Design review of the part built by this model. Coordinates are the model's own, in mm. Coordinates: 2 decimals unless noted, no trailing zeros. Write each loop counter-clockwise with the first axis right and the second up, starting at its lowest first coordinate (ties: lowest second). Pieces come first, ordered by that corner, then holes. Notation, with made-up numbers: (6, 82.25) -> (51, 82.25) arc R14 cw to (51, 109.25) -> close; hole circle Ø1 at (30, 88.25). An arc over 180 degrees is marked (long way). Return JSON: item names as keys, results as strings. Group by question number.
Autodesk Inventor part; units mm, degrees
ref_plane "YZ Plane" through (0, 0, 0) normal (1, 0, 0) x (0, 1, 0)
ref_plane "XZ Plane" through (0, 0, 0) normal (0, 1, 0) x (-1, 0, 0)
ref_plane "XY Plane" through (0, 0, 0) normal (0, 0, 1) x (1, 0, 0)
sketch "Boceto1" plane through (0, 0, 0) normal (0, 1, 0) x (-1, 0, 0)
  line L0 (0, 0) -> (80, 0)
  line L1 (80, 0) -> (80, 35)
  line L2 (80, 35) -> (0, 35)
  line L3 (0, 35) -> (0, 0)
  line L4 (75, 35) -> (5, 35)
  line L5 (5, 35) -> (5, 5)
  line L6 (5, 5) -> (75, 5)
  line L7 (75, 5) -> (75, 35)
  dimension "d0" = 80
  dimension "d1" = 35
  dimension "d2" = 70
  dimension "d3" = 30
  dimension "d14" = 5
extrude "Extrusión1" add sketch "Boceto1" along normal blind 30 contours L3 L2 L5 L6 L7 L1 L0
sketch "Boceto2" plane through (-75, 0, 5) normal (0, 0, 1) x (1, 0, 0)
  circle A0 centre (35, 15) radius 10
  point P0 (75, 0)
  dimension "d6" = 20
extrude "Extrusión2" cut sketch "Boceto2" against normal blind 30
sketch "Boceto3" plane through (-75, 0, 5) normal (1, 0, 0) x (0, 0, -1)
  circle A0 centre (-22, 15) radius 2.5
  line L0 (-30, 0) -> (-30, 30)
  line L1 (-30, 30) -> (0, 30)
  point P0 (5, 0)
  dimension "d9" = 5
  dimension "d12" = 8
  dimension "d13" = 15
extrude "Extrusión3" add sketch "Boceto3" along normal blind 70
properties part number "encaje"
Q1. Wall thickness on L1, parallel to X at y = 2.25, z = 10.5; L2, parallel to Y at x = -40, z = 1.2; L3, parallel to Z at x = -68, y = 19: over which ranges is each line inside the solid? List them lowest first.
Q2. We need section B-B on z = 16. Write out the cut boundary in (x, y).
Q3. We need section D-D on z = 27. Write out the cut boundary in (x, y), plus the area to 3 significant figures.
Q4. For P1, Ø15, axis at y = 15.5, z = 13, coming from the +X side; P2, Ø1.5, axis at x = -49.5, y = 15, coming from the +Z side; P3, Ø6, axis at x = -34.5, z = 19, coming from the +Y side; P4, Ø5, axis at x = -31.5, y = 21.5, coming from the +Z side, all flat-tipped, find the tip position at first contact; note any pin that passes through.
Q5. The part is to be moulded in two halves that separate along X. For faces 1 (the flat face through (0, 15, 18)), 2 (the cylindrical face through (-50, 15, 3)), 3 (the flat face through (-3, 15, 35)), 4 (the cylindrical face through (-40.5, 16.5, 29)), say which applies: +X half, -X half, draft (parallel to the pull), parting line (faces both ways), or undercut.
Q6. We need section C-C on y = 21. Write out the cut boundary in (x, z), plus the area to 3 significant figures.
Q7. We need section A-A on x = -40. Write out the cut boundary in (y, z), plus the area to 3 significant figures.
Findings below:
{
 "1": {"L1": "x = -80 to -75, -5 to 0", "L2": "y = 0 to 5, 25 to 30", "L3": "z = 0 to 5"},
 "2": {"outline": "(-80, 0) -> (-75, 0) -> (-75, 30) -> (-80, 30) -> close; (-5, 0) -> (0, 0) -> (0, 30) -> (-5, 30) -> close"},
 "3": {"outline": "(-80, 0) -> (-75, 0) -> (-75, 12.5) -> (-5, 12.5) -> (-5, 0) -> (0, 0) -> (0, 30) -> (-5, 30) -> (-5, 17.5) -> (-75, 17.5) -> (-75, 30) -> (-80, 30) -> close", "area": "650 mm^2"},
 "4": {"P1": "stops at x = 0", "P2": "stops at z = 29.5", "P3": "passes through", "P4": "stops at z = 5"},
 "5": {"face 1": "+X half", "face 2": "undercut", "face 3": "draft", "face 4": "undercut"},
 "6": {"outline": "(-80, 0) -> (-48, 0) -> (-48, 5) -> (-75, 5) -> (-75, 35) -> (-80, 35) -> close; (-32, 0) -> (0, 0) -> (0, 35) -> (-5, 35) -> (-5, 5) -> (-32, 5) -> close", "area": "620 mm^2"},
 "7": {"outline": "(0, 0) -> (5, 0) -> (5, 5) -> (0, 5) -> close; circle Ø5 at (15, 27); (25, 0) -> (30, 0) -> (30, 5) -> (25, 5) -> close", "area": "69.6 mm^2"}
}
